Autodesk Inventor part; units mm, degrees
ref_plane "YZ Plane" through (0, 0, 0) normal (1, 0, 0) x (0, 1, 0)
ref_plane "XZ Plane" through (0, 0, 0) normal (0, 1, 0) x (-1, 0, 0)
ref_plane "XY Plane" through (0, 0, 0) normal (0, 0, 1) x (1, 0, 0)
sketch "スケッチ1" plane through (0, 0, 0) normal (0, 0, 1) x (1, 0, 0)
  line L0 (0, 0) -> (-25, 0)
  line L1 (-25, 0) -> (-25, 30)
  line L2 (-25, 30) -> (0, 30)
  line L3 (0, 30) -> (0, 0)
  circle A0 centre (-10, 22.5) radius 1.25
  circle A1 centre (-10, 7.5) radius 1.25
  line L4 (-10, 30) -> (-10, 0)
  circle A2 centre (-10, 22.5) radius 3.25
  circle A3 centre (-10, 7.5) radius 3.25
  line L5 (-23.5, 28.5) -> (-1.5, 28.5) construction
  line L6 (-23.5, 27) -> (-1.5, 27)
  line L7 (-1.5, 30) -> (-23.5, 30)
  arc A4 (-23.5, 30) -> (-23.5, 27) centre (-23.5, 28.5) ccw
  arc A5 (-1.5, 27) -> (-1.5, 30) centre (-1.5, 28.5) ccw
  line L8 (-23.5, 1.5) -> (-1.5, 1.5) construction
  line L9 (-23.5, 0) -> (-1.5, 0)
  line L10 (-1.5, 3) -> (-23.5, 3)
  arc A6 (-23.5, 3) -> (-23.5, 0) centre (-23.5, 1.5) ccw
  arc A7 (-1.5, 0) -> (-1.5, 3) centre (-1.5, 1.5) ccw
  line L11 (-10, 28.5) -> (-10, 1.5) construction
  line L12 (-11.5, 28.5) -> (-11.5, 1.5)
  line L13 (-8.5, 1.5) -> (-8.5, 28.5)
  arc A8 (-8.5, 28.5) -> (-11.5, 28.5) centre (-10, 28.5) ccw
  arc A9 (-11.5, 1.5) -> (-8.5, 1.5) centre (-10, 1.5) ccw
  point P0 (-12.5, 28.5)
  point P1 (-12.5, 1.5)
  point P2 (-10, 15)
  point P3 (-11.5, 4.6169)
  point P4 (-11.5, 3)
  point P5 (-1.5, 0)
  point P6 (-8.5, 3)
  point P7 (-8.5, 4.6169)
  point P8 (-8.5, 10.3831)
  point P9 (-8.5, 19.6169)
  point P10 (-8.5, 25.3831)
  point P11 (-8.5, 27)
  point P12 (-11.5, 27)
  point P13 (-11.5, 25.3831)
  point P14 (-11.5, 19.6169)
  point P15 (-11.5, 10.3831)
  dimension "d0" = 25
  dimension "d1" = 30
  dimension "d2" = 2.5
  dimension "d3" = 2.5
  dimension "d4" = 10
  dimension "d5" = 15
  dimension "d6" = 2
  dimension "d7" = 2
  dimension "d8" = 3
  dimension "d9" = 3
  dimension "d10" = 3
  dimension "d11" = 6
extrude "押し出し1" add sketch "スケッチ1" along normal blind 6 contours L0 A9 L13 L10 A7 | A9 L12 L10 L4 | L0 A6 L10 L12 A9 | L4 L10 L13 A9 | A5 L6 L13 A8 L2 | L10 L12 A3 L4 | L4 A3 L13 L10 | A3 L12 L4 A1 | L4 A1 A3 L13 | L13 A2 L4 L6 | L6 L4 A8 L13 | A8 L12 L6 A4 L2 | L4 L6 L12 A8 | L13 A3 | A3 L12 | L4 A2 L12 L6 | L13 A2 L4 A0 | A2 L13 | A3 L4 A2 L13 | L12 A2 L4 A3 | L4 A0 A2 L12 | A2 L12
fillet "フィレット1" radius 1.05 12 edges at (-11.5, 25.3831, 3) (-11.5, 27, 3) (-11.5, 19.6169, 3) (-8.5, 27, 3) (-8.5, 25.3831, 3) (-8.5, 19.6169, 3) (-8.5, 10.3831, 3) (-8.5, 4.6169, 3) (-11.5, 4.6169, 3) (-11.5, 10.3831, 3) (-11.5, 3, 3) (-8.5, 3, 3)
thread "ねじ1"
thread "ねじ2"
sketch "スケッチ2" plane through (-23.5, 30, 0) normal (0, 1, 0) x (1, 0, 0)
  line L0 (22, 0) -> (0, 0)
  line L1 (0, 0) -> (0, -6)
  line L2 (22, -6) -> (0, -6)
  line L3 (22, 0) -> (22, -6)
  circle A0 centre (2.5, -2.5) radius 2.5
  line L4 (22, 0) -> (0, 0)
  line L5 (0, 0) -> (0, -6)
  circle A1 centre (19.5, -2.5) radius 2.5
  line L6 (22, 0) -> (22, -6)
  circle A2 centre (2.5, -2.5) radius 1.25
  circle A3 centre (19.5, -2.5) radius 1.25
  point P0 (23.5, 0)
  dimension "d19" = 5
  dimension "d20" = 5
  dimension "d21" = 2.5
  dimension "d22" = 2.5
extrude "押し出し2" cut sketch "スケッチ2" against normal blind 30 contours A2 | A3
thread "ねじ3"
thread "ねじ4"
thread "ねじ5"
thread "ねじ6"
properties part number "ウィング土台" material "アルミニウム 7075"
Can you work these out from the model? Positions are in its coordinate system, mm. A direction names the side the tool comes from. Give positions to 0.01 mm unless a question says otherwise; leave off trailing zeros. Order: outer loops, then holes, each group sorted by start corner. A loop starts at its lowest first (then second) coordinate and runs counter-clockwise, first axis right, second up. Notation, with made-up numbers: M -27.75,84 L -19.75,84 A22 ccw -19.75,97 Z; hole C 67.5,-34.75 d2. An arc over 180 degrees is marked long. Write item = value, one per line. Start each with the question number.
Q1. I need wall thicknesses on probe 1 along Y at (x, z) = (-10, 3.7); probe 2 along X at (y, z) = (7.5, 2.7); probe 3 along Y at (x, z) = (-5.5, 3.25). Which ranges of each line are inside material? Lowest first, please. Write a range as [from, to].
Q2. For faces 1 (the flat face through (-11, 14, 6)), 2 (the flat face through (-8.5, 15, 3)), 3 (the cylindrical face through (-11.61, 19.51, 3.04)), which set-ups out of +Z, -Z, +X, -X, +Y, -Y let a thin tool reach every point of the face, with its end or its side?
Q3. Suppose I cut it at A-A (x = -4). Write out the boundary of the cut face in (y, z).
Q4. We'd pull the mould along Y, two halves only. Please class faces 4 (the flat face through (-12, 0, 3)), 5 (the cylindrical face through (-4.921, 28.521, 1.655)), 6 (the cylindrical face through (-13.25, 22.45, 2.96)): pulls with the +Y half, pulls with the -Y half, needs draft (parallel to the pull), parting line crosses it, or undercut.
Q5. Suppose I cut it at C-C (y = 28.5). Write out the boundary of the cut face in (x, z).
Q6. Suppose I cut it at B-B (x = -10). Write out the boundary of the cut face in (y, z), plus the area to 3 significant figures.
Q7. Will these pins go through, and if not, where does the flat tip stop? pin 1 Ø3 at (y, z) = (6, 4) entering from +X; pin 2 Ø1 at (y, z) = (27, 1.5) entering from +X; pin 3 Ø3 at (y, z) = (15.5, 3) entering from -X.
Q8. Suppose I cut it at D-D (z = 3.25). Count the separate pieces of the cut face and the enclosed holes in it, plus the area to 3 significant figures.
Check result:
q1.probe_1 = [0, 6.25], [8.75, 21.25], [23.75, 30]
q1.probe_2 = [-13.25, -11.25], [-8.75, -6.75]
q1.probe_3 = [0, 3], [27, 30]
q2.face_1 = +Z, +X, -X, +Y, -Y
q2.face_2 = +Z, -Z, +X
q2.face_3 = +Z, -Z, -X
q3.outline = M 0,0 L 3,0 L 3,1.25 L 0,1.25 Z; M 0,3.75 L 3,3.75 L 3,6 L 0,6 Z; M 27,0 L 30,0 L 30,1.25 L 27,1.25 Z; M 27,3.75 L 30,3.75 L 30,6 L 27,6 Z
q4.face_4 = pulls with the -Y half
q4.face_5 = needs draft
q4.face_6 = undercut
q5.outline = M -25,0 L 0,0 L 0,6 L -25,6 Z; hole C -21,2.5 d2.5; hole C -4,2.5 d2.5
q6.outline = M 0,0 L 6.25,0 L 6.25,6 L 0,6 Z; M 8.75,0 L 21.25,0 L 21.25,6 L 8.75,6 Z; M 23.75,0 L 30,0 L 30,6 L 23.75,6 Z
q6.area = 150 mm2
q7.pin_1 = -6.75
q7.pin_2 = -0.38
q7.pin_3 = -11.5
q8.separate_pieces = 5
q8.enclosed_holes = 2
q8.area = 215 mm2
